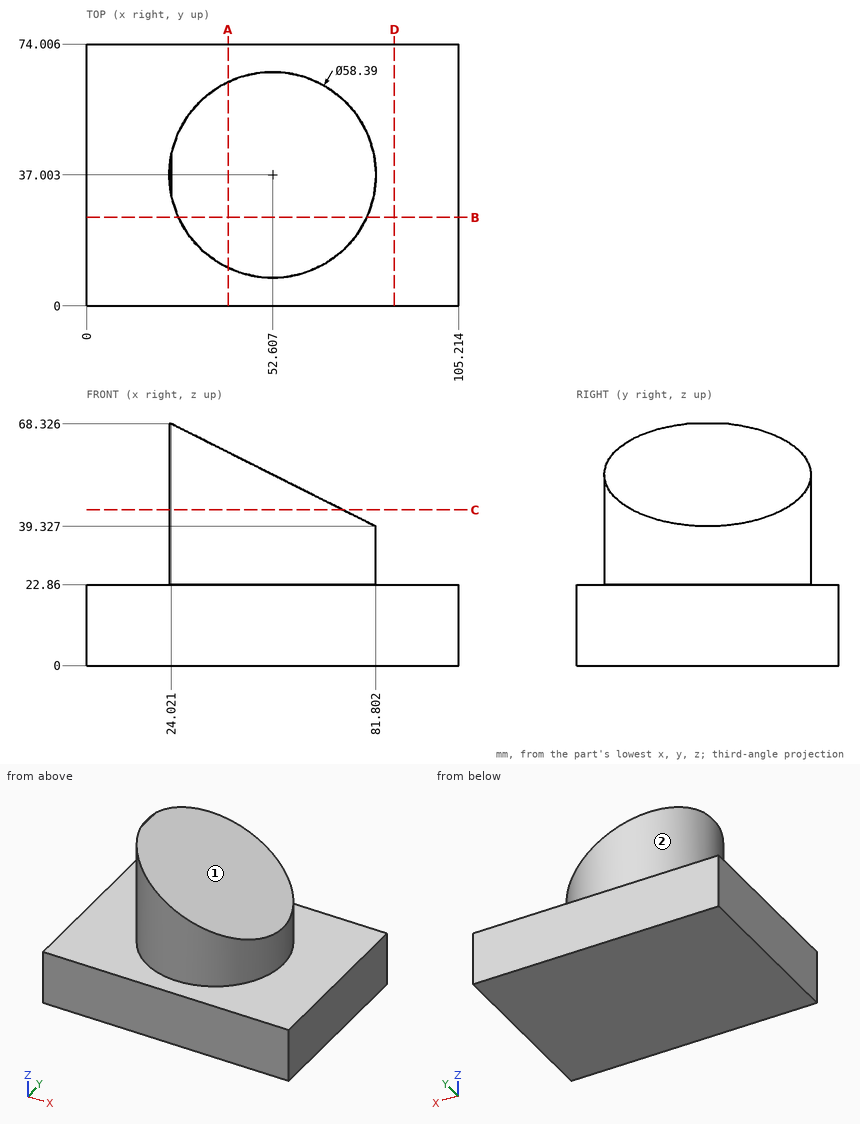
Geometry: see drawing. Coordinates: mm, zero at the bounding-box minimum. A direction names the side the tool comes from. Give positions to 0.01 mm unless a question says otherwise; leave off trailing zeros. Order: outer loops, then holes, each group sorted by start corner. A loop starts at its lowest first (then second) coordinate and runs counter-clockwise, first axis right, second up. Notation, with made-up numbers: M 31.25,-10 L 76.25,-10 A19 ccw 76.25,26 Z; hole C 74.25,-5 d6. An arc over 180 degrees is marked long. Answer as a JSON object with one key per item and string values.
1. First-contact query: P1, Ø1.5, axis at y = 19.5, z = 56.5, coming from the -X side; P2, Ø8, axis at y = 47, z = 52, coming from the +X side; P3, Ø6, axis at x = 31.5, z = 59, coming from the -Y side. Flat tips, straight axial feed; report the tip coordinate or a pass-through.
Result sheet:
{"P1": "x = 28.7", "P2": "x = 64.52", "P3": "y = 14.1"}
2. Cut plane C-C, the plane z = 44. Output: boundary loops of the cut face in (x, y) (1 decimal), and give its area (3 significant figures).
Result sheet:
{"outline": "M 72.5,15.6 L 72.5,58.4 A29.2 ccw long Z", "area": "2,400 mm²"}
3. Cut plane D-D, the plane x = 87. Output: boundary loops of the cut face in (y, z), and give its area (3 significant figures).
Result sheet:
{"outline": "M 0,0 L 74.01,0 L 74.01,22.86 L 0,22.86 Z", "area": "1,690 mm²"}
4. Reachability of the marked faces 1 and 2 from +Z, -Z, +X, -X, +Y, -Y: full face, straight path, thin tool, end or side. Return the list, or none.
Result sheet:
{"face 1": "+Z, +X, +Y, -Y", "face 2": "+Z"}
5. Ray query, line 1 (Z direction, x = 94, y = 34.5); line 2 (X direction, y = 37.5, z = 29.5); line 3 (Y direction, x = 43, z = 52.5) (1 decimal). Return the intervals inside material, ascending. Write a range as [from, to].
Result sheet:
{"line 1": "[0, 22.86]", "line 2": "[23.42, 81.8]", "line 3": "[9.4, 64.6]"}
6. Cut plane A-A, the plane x = 40. Output: boundary loops of the cut face in (y, z) (1 decimal), and give its area (3 significant figures).
Result sheet:
{"outline": "M 0,0 L 74,0 L 74,22.9 L 63.3,22.9 L 63.3,60.3 L 10.7,60.3 L 10.7,22.9 L 0,22.9 Z", "area": "3,660 mm²"}
7. Cut plane B-B, the plane y = 25. Output: boundary loops of the cut face in (x, z).
Result sheet:
{"outline": "M 0,0 L 105.21,0 L 105.21,22.86 L 79.22,22.86 L 79.22,40.62 L 25.99,67.34 L 25.99,22.86 L 0,22.86 Z"}
